```python
from build123d import *

# Parameters (mm, degrees)
F0_W      = 50
F0_H      = 50
F1_DEPTH  = 5
F2_W      = 40
F2_H      = 45
F3_DEPTH  = 5.001
F4_R      = 5
F6_DEPTH  = 5
F8_DEPTH  = 5.001
F10_DEPTH = 5
F12_DEPTH = 5.001


# Not quite as in the source:
# - ends of sketch curves that miss each other by under 0.0002 mm in the source are joined


with BuildPart() as f1:
    # F0 (on Top) → F1 (new body)
    with BuildSketch(Plane.XY):
        Rectangle(F0_W, F0_H)
    extrude(amount=F1_DEPTH)

    # F2 (on face) → F3 (cut, through all)
    with BuildSketch(Plane.XY.offset(5)):
        with Locations((0, -2.5)):
            Rectangle(F2_W, F2_H)
    extrude(amount=-F3_DEPTH, mode=Mode.SUBTRACT)

    # F4
    f4_edges = [f1.edges().sort_by_distance(p)[0] for p in [
        (-20, 20, 2.5),
        (20, 20, 2.5),
        (25, 25, 2.5),
        (-25, 25, 2.5),
    ]]
    fillet(f4_edges, radius=F4_R)

    # F5 (on face) → F6 (join)
    with BuildSketch(Plane.XY.offset(5)):
        Polygon((-25, -19.9999040991), (-25, -15), (-30, -15), align=None)
    extrude(amount=-F6_DEPTH)

    # F7 (on face) → F8 (cut, through all)
    with BuildSketch(Plane.XY.offset(5)):
        Polygon((-20, -25), (-25.0000479505, -19.9999520495), (-25, -25), align=None)
    extrude(amount=-F8_DEPTH, mode=Mode.SUBTRACT)

    # F9 (on Top) → F10 (join)
    with BuildSketch(Plane.XY):
        Polygon((30, -15), (25, -15), (25, -20), align=None)
    extrude(amount=F10_DEPTH)

    # F11 (on face) → F12 (cut, through all)
    with BuildSketch(Plane.XY.offset(5)):
        Polygon((25, -25), (25, -20), (20, -25), align=None)
    extrude(amount=-F12_DEPTH, mode=Mode.SUBTRACT)


solid = f1.part
```
Here's how the part is built. I have some questions about the finished solid (model axes, mm). A direction names the side the tool comes from. Round coordinates to 2 decimals unless told otherwise and drop trailing zeros. Write each loop counter-clockwise with the first axis right and the second up, starting at its lowest first coordinate (ties: lowest second). Pieces come first, ordered by that corner, then holes.
Q1. If we section it at A-A on y = 2: Write out the boundary of the cut face in (x, z).
Q2. Will these pins go through, and if not, where does the flat tip stop? P1, Ø1.5, axis at x = 17.5, y = 7, coming from the -Z side; P2, Ø1.5, axis at y = -2.5, z = 1.5, coming from the +X side; P3, Ø2.5, axis at y = 2.5, z = 3.5, coming from the -X side; P4, Ø1.5, axis at x = 28.5, z = 3.5, coming from the +Y side.
Q3. If we section it at C-C on y = 18.5: Write out the boundary of the cut face in (x, z).
Q4. If we mould it in two halves opening along X, with no side actions, what happens to faces 6 (the flat face through (0, 20, 3)), 7 (the flat face through (25, 2, 2)), 8 (the flat face through (-28, -17, 3)), 9 (the flat face through (-20, -5, 3))? For each: +X half, -X half, draft (parallel to the pull), parting line (faces both ways), or undercut.
Q5. Which directions (+Z, -Z, +X, -X, +Y, -Y) give clear straight access to the entire face, cutting with the end or side of a thin tool? Please do faces 1 (the flat face through (-22, -23, 3)), 2 (the flat face through (-4.6, 20.5, 0)), 3 (the cylindrical face through (19, 18, 2)), 4 (the flat face through (-27, -15, 3)), 5 (the flat face through (28, -15, 2)).
Q6. If we section it at D-D on x = -9: Write out the boundary of the cut face in (y, z), plus the area to 3 significant figures.
Q7. Please list where these lines run through material, in increasing order: probe 1 along X at (y, z) = (7, 2.55); probe 2 along Y at (x, z) = (-10, 2.7); probe 3 along X at (y, z) = (-21, 2.65).
Answer below:
1. outline: (-25, 0) - (-20, 0) - (-20, 5) - (-25, 5) - close; (20, 0) - (25, 0) - (25, 5) - (20, 5) - close
2. P1: passes through
2. P2: stops at x = 25
2. P3: stops at x = -25
2. P4: stops at y = -15
3. outline: (-25, 0) - (-18.57, 0) - (-18.57, 5) - (-25, 5) - close; (18.57, 0) - (25, 0) - (25, 5) - (18.57, 5) - close
4. face 6: undercut
4. face 7: +X half
4. face 8: -X half
4. face 9: undercut
5. face 1: +Z, -Z, -X, -Y
5. face 2: -Z, +X, -X, +Y, -Y
5. face 3: +Z, -Z, -Y
5. face 4: +Z, -Z, -X, +Y
5. face 5: +Z, -Z, +X, +Y
6. outline: (20, 0) - (25, 0) - (25, 5) - (20, 5) - close
6. area: 25.0 mm2
7. probe 1: x = -25 to -20, 20 to 25
7. probe 2: y = 20 to 25
7. probe 3: x = -24 to -20, 20 to 24
